```python
from build123d import *

# Parameters (mm, degrees)
BOSS_EXTRUDE1_DEPTH = 70
CHAMFER1_SIZE       = 40
CHAMFER1_SIZE2      = 3.7
CHAMFER2_SIZE       = 3.7
CHAMFER2_SIZE2      = 40


with BuildPart() as part:
    # Sketch1 → Boss-Extrude1 (new body)
    with BuildSketch(Plane.XY):
        Polygon((0, 0), (0, 55), (3, 55), (3, 45), (15.4, 45), (15.4, 55), (18.4, 55), (18.4, 0), (11.7, 0), (11.7, 5), (6.7, 5), (6.7, 0), align=None)
    extrude(amount=BOSS_EXTRUDE1_DEPTH)

    # Chamfer1
    chamfer1_edges = [part.edges().sort_by_distance(p)[0] for p in [
        (0, 0, 35),
    ]]
    chamfer1_side = [part.faces().sort_by_distance(p)[0] for p in [
        (0, 27.5, 35),
    ]]
    chamfer(chamfer1_edges, length=CHAMFER1_SIZE, length2=CHAMFER1_SIZE2, reference=chamfer1_side[0])

    # Chamfer2
    chamfer2_edges = [part.edges().sort_by_distance(p)[0] for p in [
        (18.4, 0, 35),
    ]]
    chamfer2_side = [part.faces().sort_by_distance(p)[0] for p in [
        (15.05, 0, 35),
    ]]
    chamfer(chamfer2_edges, length=CHAMFER2_SIZE, length2=CHAMFER2_SIZE2, reference=chamfer2_side[0])


solid = part.part
```
Work out the finished part from the listing and answer in its coordinate system (mm). A direction names the side the tool comes from. Give positions to 0.01 mm unless a question says otherwise; leave off trailing zeros. Order: outer loops, then holes, each group sorted by start corner. A loop starts at its lowest first (then second) coordinate and runs counter-clockwise, first axis right, second up.
1. Section A-A, the plane y = 46.5 is taken. Determine the outline of the cut face in (x, z), and give its area (3 significant figures).
Result sheet:
outline: (0, 0) - (3, 0) - (3, 70) - (0, 70) - close; (15.4, 0) - (18.4, 0) - (18.4, 70) - (15.4, 70) - close
area: 420 mm2
2. For faces 4 (the flat face through (6.7, 3, 35)), 5 (the flat face through (9, 45, 35)), 6 (the flat face through (5, 0, 35)), determine the directions among +Z, -Z, +X, -X, +Y, -Y from which every point of the face is accessible in a straight line to the end or side of a thin tool.
Result sheet:
face 4: +Z, -Z, -Y
face 5: +Z, -Z, +Y
face 6: +Z, -Z, +X, -X, -Y
3. Straight lines are drawn through the part: L1, parallel to X at y = 48.5, z = 5; L2, parallel to Y at x = 4, z = 51.5; L3, parallel to Y at x = 9.75, z = 42. For each, find the intervals that lie inside material, in ascending order.
Result sheet:
L1: x = 0 to 3, 15.4 to 18.4
L2: y = 0 to 45
L3: y = 5 to 45
4. Each of these flat-tipped pins is pushed along its axis until it touches: P1, Ø3.5, axis at x = 10.5, z = 41, coming from the +Y side; P2, Ø8, axis at y = 21, z = 44.5, coming from the -X side; P3, Ø4, axis at x = 9, z = 23.5, coming from the -Y side. Where does it stop, or does it pass through?
Result sheet:
P1: stops at y = 45
P2: stops at x = 1.39
P3: stops at y = 5
5. Section B-B, the plane z = 48 is taken. Determine the outline of the cut face in (x, y).
Result sheet:
outline: (0, 40) - (3.7, 0) - (6.7, 0) - (6.7, 5) - (11.7, 5) - (11.7, 0) - (14.7, 0) - (18.4, 40) - (18.4, 55) - (15.4, 55) - (15.4, 45) - (3, 45) - (3, 55) - (0, 55) - close
6. Section D-D, the plane y = 28 is taken. Determine the outline of the cut face in (x, z).
Result sheet:
outline: (1.11, 0) - (17.29, 0) - (17.29, 70) - (1.11, 70) - close
7. Section C-C, the plane x = 8.25 is taken. Determine the outline of the cut face in (y, z), and give its area (3 significant figures).
Result sheet:
outline: (5, 0) - (45, 0) - (45, 70) - (5, 70) - close
area: 2,800 mm2
8. The mould has two halves that part along X. Classify faces 1 (the flat face through (0, 47, 35)), 2 (the flat face through (18.4, 48, 35)), 3 (the flat face through (15.4, 50, 35)): released by +X, released by -X, zero draft, split by the parting line, or undercut.
Result sheet:
face 1: released by -X
face 2: released by +X
face 3: undercut
